Answer from the drawing. Dimensions are ordinates in mm from the lowest x, y and z of the part. A direction names the side the tool comes from. Give positions to 0.01 mm unless a question says otherwise; leave off trailing zeros. Write each loop counter-clockwise with the first axis right and the second up, starting at its lowest first coordinate (ties: lowest second). Pieces come first, ordered by that corner, then holes.
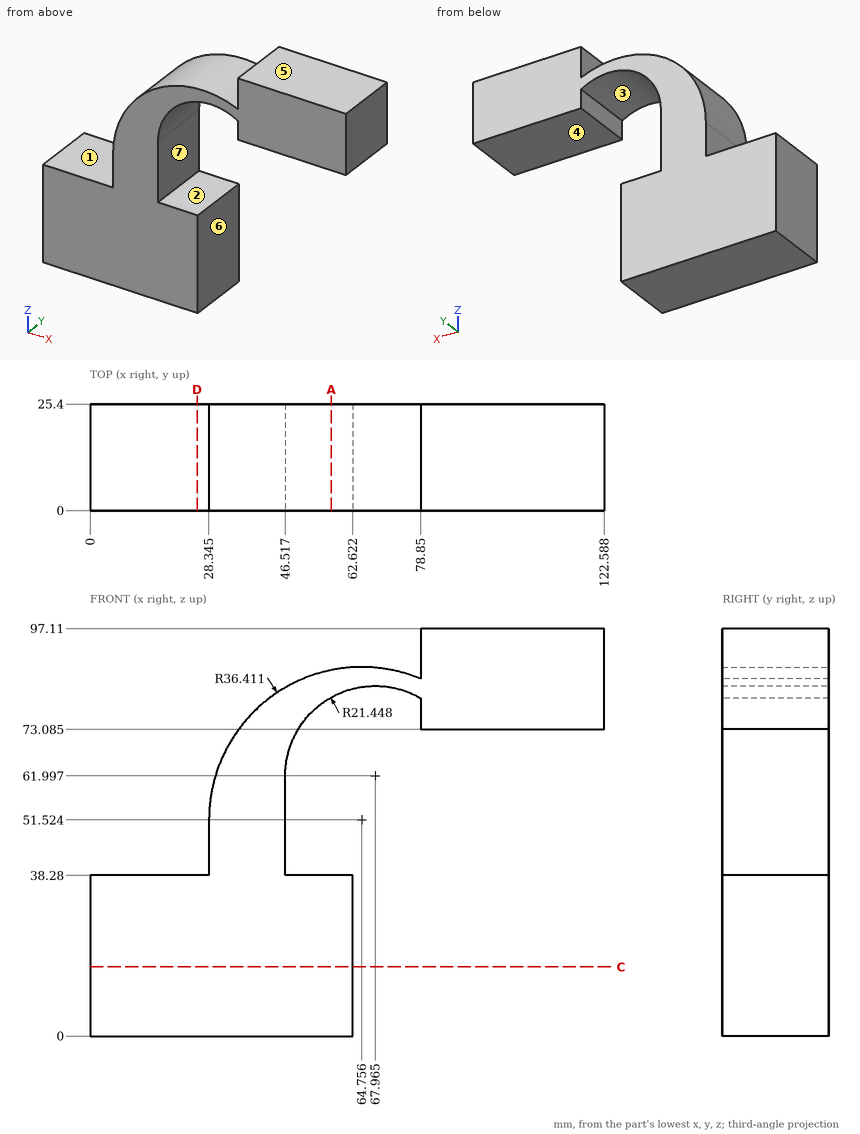
Item 1: A cutting plane is placed at A-A, the plane x = 57.5. Give the vertices of the cut face in (y, z) (1 decimal), plus the area to 3 significant figures.
Conclusion:
outline: (0, 0) - (25.4, 0) - (25.4, 38.3) - (0, 38.3) - close; (0, 80.7) - (25.4, 80.7) - (25.4, 87.2) - (0, 87.2) - close
area: 1,140 mm2
Item 2: A cutting plane is placed at C-C, the plane z = 16.5. Give the vertices of the cut face in (x, y), plus the area to 3 significant figures.
Conclusion:
outline: (0, 0) - (62.62, 0) - (62.62, 25.4) - (0, 25.4) - close
area: 1,590 mm2
Item 3: Consider probe 1 along Z at (x, y) = (25, 20.25); probe 2 along X at (y, z) = (18.25, 74); probe 3 along X at (y, z) = (8.75, 49.5) (1 decimal). Determine where each line is inside the solid, lowest interval first.
Conclusion:
probe 1: z = 0 to 38.28
probe 2: x = 36.11 to 50.19, 78.85 to 122.59
probe 3: x = 28.3 to 46.5
Item 4: Determine the mould class of the marked faces 5, 6 and 7 for opening direction Z: pulls with the +Z half, pulls with the -Z half, needs draft (parallel to the pull), parting line crosses it, or undercut.
Conclusion:
face 5: pulls with the +Z half
face 6: needs draft
face 7: undercut
Item 5: Each of these flat-tipped pins is pushed along its axis until it touches: P1, Ø1, axis at y = 9.5, z = 13.5, coming from the +X side; P2, Ø8, axis at y = 8.5, z = 87, coming from the -X side; P3, Ø12, axis at x = 43.5, y = 7, coming from the +Z side (1 decimal). Where does it stop, or does it pass through?
Conclusion:
P1: stops at x = 62.62
P2: stops at x = 46.45
P3: stops at z = 84.6
Item 6: A cutting plane is placed at D-D, the plane x = 25.5. Give the vertices of the cut face in (y, z).
Conclusion:
outline: (0, 0) - (25.4, 0) - (25.4, 38.28) - (0, 38.28) - close
Item 7: Which of the six approach directions +Z, -Z, +X, -X, +Y, -Y give full straight-line access (tool end or side, diameter ignored) to the marked faces 1, 2, 3 and 4?
Conclusion:
face 1: +Z, -X, +Y, -Y
face 2: +X, +Y, -Y
face 3: +Y, -Y
face 4: -Z, +X, +Y, -Y
